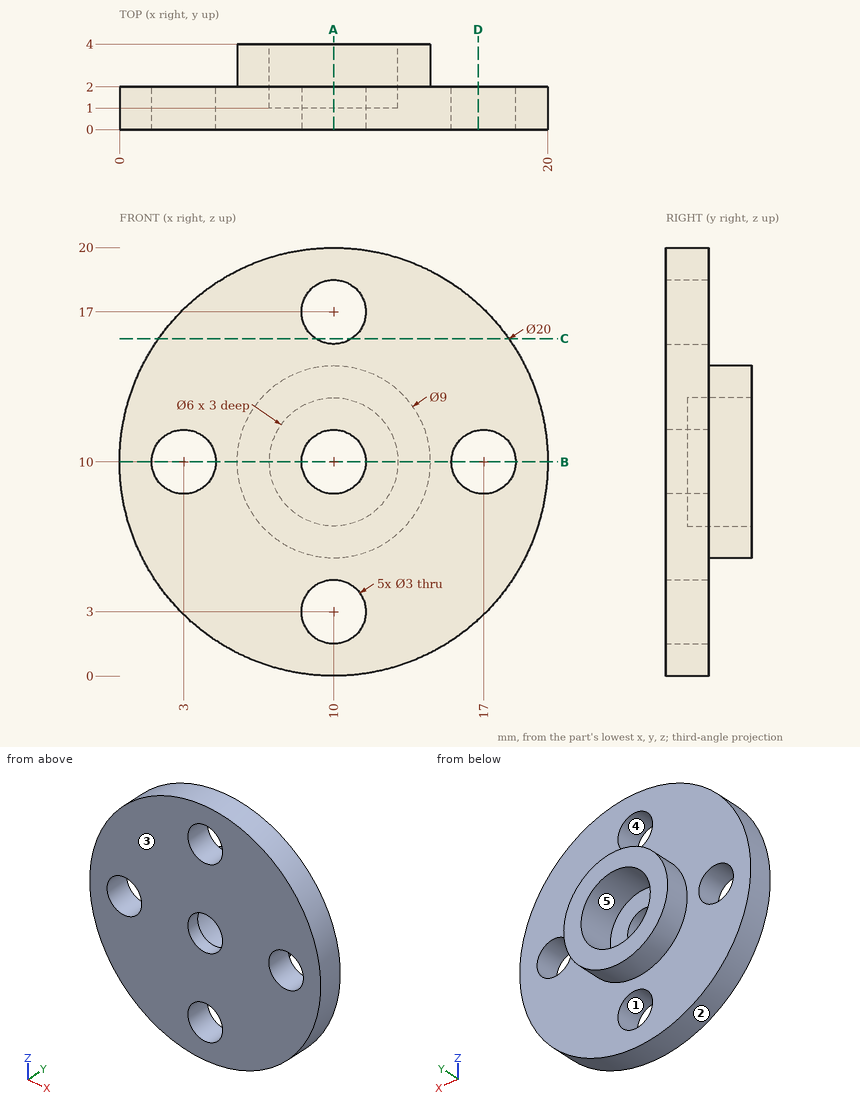
Could you check a few things on this drawing? It's one solid part, dimensions in mm from its lowest x, y, z. A direction names the side the tool comes from. Round coordinates to 2 decimals unless told otherwise and drop trailing zeros. Loops run counter-clockwise (first coordinate to the right, second up) from the corner with the lowest first, then second, coordinate; pieces in that order, holes last.
Q1. I want a section at A-A (x = 10). Write out the boundary of the cut face in (y, z), and give its area (3 significant figures).
Q2. For P1, Ø2.5, axis at x = 10, z = 3, coming from the -Y side; P2, Ø1, axis at x = 13.5, y = 1.5, coming from the +Z side, each with a flat end and sliding along its axis, tell me the tip position at first contact or that it passes through.
Q3. I want a section at C-C (z = 15.75). Write out the boundary of the cut face in (x, y), and give its area (3 significant figures).
Q4. I want a section at B-B (z = 10). Write out the boundary of the cut face in (x, y), and give its area (3 significant figures).
Q5. On a 3-axis mill with a long thin cutter (end or side, diameter ignored), from which of +Z, -Z, +X, -X, +Y, -Y can I reach the whole of each face in a straight line? I mean the marked faces 4 and 5. Say none if no direction works.
Q6. Please list where these lines run through material, in increasing order: L1, parallel to X at y = 1.95, z = 10; L2, parallel to X at y = 0.7, z = 10; L3, parallel to X at y = 2.65, z = 10.
Q7. I want a section at D-D (x = 16.75). Write out the boundary of the cut face in (y, z).
Q8. Thinking about a two-plate mould opening in Z: for the marked faces 1, 2 and 3, which applies, pulls with the +Z half, pulls with the -Z half, needs draft (parallel to the pull), parting line crosses it, or undercut?
Answer below:
1. outline: (0, 0) - (2, 0) - (2, 1.5) - (0, 1.5) - close; (0, 4.5) - (2, 4.5) - (2, 5.5) - (4, 5.5) - (4, 7) - (1, 7) - (1, 8.5) - (0, 8.5) - close; (0, 11.5) - (1, 11.5) - (1, 13) - (4, 13) - (4, 14.5) - (2, 14.5) - (2, 15.5) - (0, 15.5) - close; (0, 18.5) - (2, 18.5) - (2, 20) - (0, 20) - close
1. area: 25.0 mm2
2. P1: passes through
2. P2: stops at z = 19.54
3. outline: (1.82, 0) - (9.17, 0) - (9.17, 2) - (1.82, 2) - close; (10.83, 0) - (18.18, 0) - (18.18, 2) - (10.83, 2) - close
3. area: 29.4 mm2
4. outline: (0, 0) - (1.5, 0) - (1.5, 2) - (0, 2) - close; (4.5, 0) - (8.5, 0) - (8.5, 1) - (7, 1) - (7, 4) - (5.5, 4) - (5.5, 2) - (4.5, 2) - close; (11.5, 0) - (15.5, 0) - (15.5, 2) - (14.5, 2) - (14.5, 4) - (13, 4) - (13, 1) - (11.5, 1) - close; (18.5, 0) - (20, 0) - (20, 2) - (18.5, 2) - close
4. area: 25.0 mm2
5. face 4: +Y, -Y
5. face 5: +Y
6. L1: x = 0 to 1.5, 4.5 to 7, 13 to 15.5, 18.5 to 20
6. L2: x = 0 to 1.5, 4.5 to 8.5, 11.5 to 15.5, 18.5 to 20
6. L3: x = 5.5 to 7, 13 to 14.5
7. outline: (0, 2.62) - (2, 2.62) - (2, 8.52) - (0, 8.52) - close; (0, 11.48) - (2, 11.48) - (2, 17.38) - (0, 17.38) - close
8. face 1: undercut
8. face 2: parting line crosses it
8. face 3: needs draft
